Model file for the job. Use its own axes, mm. Face numbers are marked on the shaded views. A direction names the side the tool comes from. Coordinates: 2 decimals unless noted, no trailing zeros. Order: outer loops, then holes, each group sorted by start corner. A loop starts at its lowest first (then second) coordinate and runs counter-clockwise, first axis right, second up. Notation, with made-up numbers: (-9, -23.75) -> (33, -23.75) arc R10 cw to (33, -9.75) -> close; hole circle Ø8 at (14, 76.25). An arc over 180 degrees is marked (long way). Write item = value, one per line. Start each with the question number.
Q1. Cut at D-D, the plane z = -18. List the corners of the cut face in (x, y), plus the area to 3 significant figures.
Q2. Cut at C-C, the plane y = -42. List the corners of the cut face in (x, z) (1 decimal).
Q3. Wall check: line 1 (Z direction, x = 0, y = -20.5); line 2 (Z direction, x = 0, y = -85) (3 decimals); line 3 (Y direction, x = 8, z = -24.5). Give the ranges that are in metal, low to high. Write a range as from..to.
Q4. 3-axis set-ups, long thin cutter, end or side, ignore diameter. For the marked faces 4 and 5: which of +Z, -Z, +X, -X, +Y, -Y reach the whole face in a straight line?
Q5. Cut at B-B, the plane x = 0. List the corners of the cut face in (y, z) (1 decimal).
Q6. Mould opens along X. For the marked faces 1, 2 and 3 say: +X half, -X half, draft (parallel to the pull), parting line (faces both ways), or undercut.
Q7. Cut at A-A, the plane z = 0. List the corners of the cut face in (x, y) (1 decimal), plus the area to 3 significant figures.
Q8. Flat gauge pins, fed straight in: pin 1 (12 mm diameter, centred on y = -20.5, z = 22, fed in from +X); pin 2 (10 mm diameter, centred on y = -77.5, z = 4.5, fed in from +X); pin 3 (22 mm diameter, centred on x = 15, z = -8, fed in from +Y); pin 4 (1 mm diameter, centred on x = 27.5, z = -28, fed in from +Y). Where does each tip first touch, or does it go through?
from build123d import *

# Parameters (mm, degrees)
F0_R     = 39.1668
F0_R_2   = 36.5125
F1_DEPTH = 45.72
F3_R     = 39.1668
F3_R_2   = 13.335
F4_DEPTH = 5.08
F6_R     = 15.9258
F6_R_2   = 13.335
F7_DEPTH = 50.8


with BuildPart() as f1:
    # F0 (on Front) → F1 (new body)
    with BuildSketch(Plane.XZ):
        Circle(F0_R)
        Circle(F0_R_2, mode=Mode.SUBTRACT)
    extrude(amount=F1_DEPTH)

    # F3 (on offset) → F4 (join)
    with BuildSketch(Plane.XZ.offset(45.72)):
        Circle(F3_R)
        Circle(F3_R_2, mode=Mode.SUBTRACT)
    extrude(amount=F4_DEPTH)

    # F6 (on offset) → F7 (join)
    with BuildSketch(Plane.XZ.offset(50.8)):
        Circle(F6_R)
        Circle(F6_R_2, mode=Mode.SUBTRACT)
    extrude(amount=F7_DEPTH)


solid = f1.part
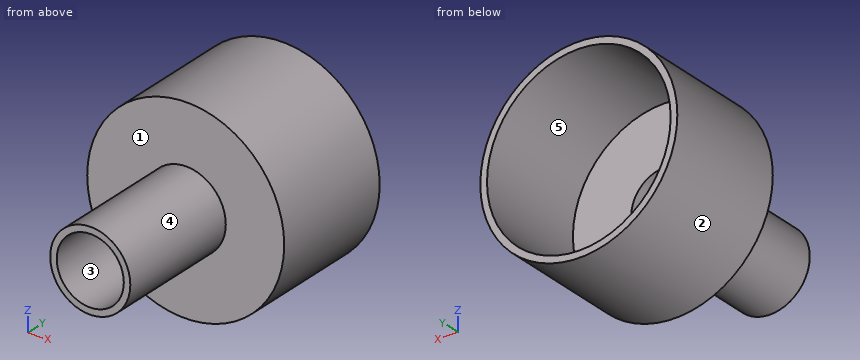
Here are the results:
q1.outline = (-34.79, -50.8) -> (34.79, -50.8) -> (34.79, 0) -> (31.77, 0) -> (31.77, -45.72) -> (-31.77, -45.72) -> (-31.77, 0) -> (-34.79, 0) -> close
q1.area = 629 mm²
q2.outline = circle Ø78.3 at (0, 0); hole circle Ø73 at (0, 0)
q3.line_1 = -39.17..-36.51, 36.51..39.17
q3.line_2 = -15.926..-13.335, 13.335..15.926
q3.line_3 = -50.8..-45.72
q4.face_4 = -Y
q4.face_5 = +Y
q5.outline = (-101.6, -15.9) -> (-50.8, -15.9) -> (-50.8, -39.2) -> (0, -39.2) -> (0, -36.5) -> (-45.7, -36.5) -> (-45.7, -13.3) -> (-101.6, -13.3) -> close; (-101.6, 13.3) -> (-45.7, 13.3) -> (-45.7, 36.5) -> (0, 36.5) -> (0, 39.2) -> (-50.8, 39.2) -> (-50.8, 15.9) -> (-101.6, 15.9) -> close
q6.face_1 = draft
q6.face_2 = parting line
q6.face_3 = undercut
q7.outline = (-39.2, -50.8) -> (-15.9, -50.8) -> (-15.9, -101.6) -> (-13.3, -101.6) -> (-13.3, -45.7) -> (-36.5, -45.7) -> (-36.5, 0) -> (-39.2, 0) -> close; (13.3, -101.6) -> (15.9, -101.6) -> (15.9, -50.8) -> (39.2, -50.8) -> (39.2, 0) -> (36.5, 0) -> (36.5, -45.7) -> (13.3, -45.7) -> close
q7.area = 768 mm²
q8.pin_1 = 35.75
q8.pin_2 = 15.93
q8.pin_3 = -45.72
q8.pin_4 = 0
